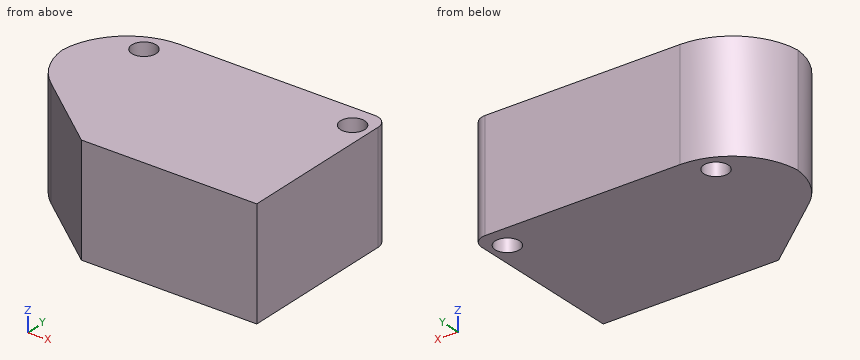
from build123d import *

# Parameters (mm, degrees)
F0_W        = 101.6
F0_H        = 39.83482
F1_DEPTH    = 63.5
F3_DEPTH    = 106.68
F4_T1_DEPTH = 101.2392583659
F4_T3_DEPTH = 166.83482
F5_R        = 5.08
F6_R        = 4.445
F7_DEPTH    = 50.8


# Not quite as in the source:
# - a fillet or chamfer that OpenCascade refuses, or shapes differently, is made with other operations: its cross-section is extruded or revolved along the edge and cut away or added


with BuildPart() as f1:
    # F0 (on Front) → F1 (new body)
    with BuildSketch(Plane.XZ):
        with Locations((-50.8, -19.91741)):
            Rectangle(F0_W, F0_H)
    extrude(amount=F1_DEPTH)

    # F2 (on face) → F3 (cut)
    with BuildSketch(Plane(origin=(0, 0, -39.83482), x_dir=(1, 0, 0), z_dir=(0, 0, -1))):
        Polygon((-101.6, 63.5), (-101.6, 33.7622053921), (-64.0701651573, 63.5), align=None)
    extrude(amount=-F3_DEPTH, mode=Mode.SUBTRACT)

    # F4: fillet of radius 25.4 on 2 edges, made by hand

    # F4_s2 → F4_t1 (cut)
    with BuildSketch(Plane.XY.offset(-70.537039183)):
        with BuildLine():
            ThreePointArc((-91.9745517237, -41.389193495), (-99.0673742894, -32.5376820901), (-101.6, -21.4813177189))
            Line((-101.6, -21.4813177189), (-101.6, -33.7622053921))
            Line((-101.6, -33.7622053921), (-91.9745517237, -41.389193495))
        make_face()
    extrude(amount=F4_T1_DEPTH, mode=Mode.SUBTRACT)

    # F4_s4 → F4_t3 (cut)
    with BuildSketch(Plane.XY.offset(-103.33482)):
        with BuildLine():
            ThreePointArc((-76.2, 0), (-94.1605122421, -7.4394877579), (-101.6, -25.4))
            Line((-101.6, -25.4), (-101.6, 0))
            Line((-101.6, 0), (-76.2, 0))
        make_face()
    extrude(amount=F4_T3_DEPTH, mode=Mode.SUBTRACT)

    # F5
    f5_edges = [f1.edges().sort_by_distance(p)[0] for p in [
        (0, 0, -19.91741),
    ]]
    fillet(f5_edges, radius=F5_R)

    # F6 (on face) → F7 (cut)
    with BuildSketch(Plane(origin=(0, 0, -39.83482), x_dir=(1, 0, 0), z_dir=(0, 0, -1))):
        with Locations((-82.8581005335, 8.6406739429)):
            Circle(F6_R)
        with Locations((-6.6581005335, 8.6406739429)):
            Circle(F6_R)
    extrude(amount=-F7_DEPTH, mode=Mode.SUBTRACT)


solid = f1.part
Geometry: final body of the model. Coordinates: model frame, mm. Give positions to 0.01 mm unless a question says otherwise; leave off trailing zeros. Order: outer loops, then holes, each group sorted by start corner. A loop starts at its lowest first (then second) coordinate and runs counter-clockwise, first axis right, second up. Notation, with made-up numbers: (-20.5, 45) -> (27.5, 45) arc R18 ccw to (27.5, 72) -> close; hole circle Ø5 at (2.5, 58.5). An arc over 180 degrees is marked (long way). Write each question's results on one line, items separated by ' | '.
1) Line query: line 1 along X through (y, z) = (-10, -2.5); line 2 along X through (y, z) = (-6, -29); line 3 along Y through (x, z) = (-82.5, -37). Output: solid intervals per line, ascending.
Geometry says:
line 1: x = -96.4 to -87.09, -78.63 to -10.89, -2.43 to 0 | line 2: x = -92.6 to -86.43, -79.28 to -10.23, -3.08 to 0 | line 3: y = -48.9 to -13.07, -4.21 to -0.79
2) Cut plane C-C (x = -8). Output: boundary loops of the cut face in (y, z), and give its area (3 significant figures).
Geometry says:
outline: (-63.5, -39.83) -> (-12.88, -39.83) -> (-12.88, 0) -> (-63.5, 0) -> close; (-4.4, -39.83) -> (0, -39.83) -> (0, 0) -> (-4.4, 0) -> close | area: 2,190 mm²
3) Cut plane A-A (y = -7.5). Output: boundary loops of the cut face in (x, z), and give its area (3 significant figures).
Geometry says:
outline: (-94.22, -39.83) -> (-87.15, -39.83) -> (-87.15, 0) -> (-94.22, 0) -> close; (-78.56, -39.83) -> (-10.95, -39.83) -> (-10.95, 0) -> (-78.56, 0) -> close; (-2.36, -39.83) -> (0, -39.83) -> (0, 0) -> (-2.36, 0) -> close | area: 3,070 mm²
4) Cut plane B-B (z = -22.5). Output: boundary loops of the cut face in (x, y) (3 decimals), and give its area (3 significant figures).
Geometry says:
outline: (-101.524, -23.441) arc R25.4 ccw to (-91.975, -41.389) -> (-64.07, -63.5) -> (0, -63.5) -> (0, -5.08) arc R5.08 ccw to (-5.08, 0) -> (-76.2, 0) arc R25.4 ccw to start; hole circle Ø8.89 at (-82.858, -8.641); hole circle Ø8.89 at (-6.658, -8.641) | area: 5,600 mm²
5) First-contact query: pin 1 Ø5.5 at (x, y) = (-6.66, -8.64) entering from -Z; pin 2 Ø3 at (x, z) = (-86.5, -27.5) entering from -Y; pin 3 Ø1 at (y, z) = (-25, -12) entering from -X; pin 4 Ø2 at (y, z) = (-9, -19.5) entering from -X. Flat tips, straight axial feed; report the tip coordinate or a pass-through.
Geometry says:
pin 1: passes through | pin 2: stops at y = -46.92 | pin 3: stops at x = -101.42 | pin 4: stops at x = -96.4
6) Cut plane D-D (y = -38). Output: boundary loops of the cut face in (x, z), and give its area (3 significant figures).
Geometry says:
outline: (-95.49, -39.83) -> (0, -39.83) -> (0, 0) -> (-95.49, 0) -> close | area: 3,800 mm²
